Autodesk Inventor part; units mm, degrees
ref_plane "YZ Plane" through (0, 0, 0) normal (1, 0, 0) x (0, 1, 0)
ref_plane "XZ Plane" through (0, 0, 0) normal (0, 1, 0) x (-1, 0, 0)
ref_plane "XY Plane" through (0, 0, 0) normal (0, 0, 1) x (1, 0, 0)
sketch "Sketch1" plane through (0, 0, 0) normal (0, 0, 1) x (1, 0, 0)
  circle A0 centre (0, 0) radius 6.5
  dimension "d0" = 13
extrude "Extrusion1" add sketch "Sketch1" along normal blind 2.5
sketch "Sketch2" plane through (0, 0, 2.5) normal (0, 0, 1) x (1, 0, 0)
  circle A0 centre (0, 0) radius 1.55
  dimension "d3" = 3.1
extrude "Extrusion2" cut sketch "Sketch2" against normal through all
sketch "Sketch3" plane through (0, 0, 0) normal (0, 0, -1) x (-1, 0, 0)
  circle A0 centre (0, 0) radius 2.96
  circle A1 centre (0, 0) radius 7.5
  dimension "d6" = 5.92
  dimension "d16" = 15
extrude "Extrusion3" cut sketch "Sketch3" against normal blind 0.8
sketch "Sketch4" plane through (0, 0, 2.5) normal (0, 0, 1) x (1, 0, 0)
  circle A0 centre (0, 0) radius 2.5
  dimension "d9" = 5
extrude "Extrusion4" cut sketch "Sketch4" against normal blind 1.5
sketch "Sketch5" plane through (0, 0, 2.5) normal (0, 0, 1) x (1, 0, 0)
  circle A0 centre (0, 0) radius 6.5
  circle A1 centre (0, 0) radius 2.5
  circle A2 centre (0, 0) radius 3.025
  circle A3 centre (0, 0) radius 6.5
  dimension "d12" = 6.05
  dimension "d15" = 0
extrude "Extrusion5" add sketch "Sketch5" along normal blind 2.5 contours A0
chamfer "Chamfer1" distance 2 angle 45 1 edges at (-6.5, 0, 0.8)
properties part number "motor_and_magnet_holder"
Work out the finished part from the listing and answer in its coordinate system (mm). A direction names the side the tool comes from. Round coordinates to 2 decimals unless told otherwise and drop trailing zeros. Write each loop counter-clockwise with the first axis right and the second up, starting at its lowest first coordinate (ties: lowest second). Pieces come first, ordered by that corner, then holes. Notation, with made-up numbers: (-20.75, 10.5) -> (21.25, 10.5) arc R26 cw to (21.25, 40.5) -> close; hole circle Ø3 at (-32.75, -25). An arc over 180 degrees is marked (long way). Write each question's results on one line, items separated by ' | '.
Item 1: Which of the six approach directions +Z, -Z, +X, -X, +Y, -Y give full straight-line access (tool end or side, diameter ignored) to faces 4 (the face through (-2, 2, 2.5)), 5 (the face through (-5.158, 3.955, 3.885)), 6 (the face through (2.35, -1.8, 0.39))?
Result set:
face 4: +Z | face 5: +Z, -Z | face 6: -Z
Item 2: A cutting plane is placed at A-A, the plane y = 0. Determine the outline of the cut face in (x, z) (3 decimals), plus the area to 3 significant figures.
Result set:
outline: (-6.5, 2.8) -> (-4.5, 0.8) -> (-2.96, 0.8) -> (-2.96, 0) -> (-1.55, 0) -> (-1.55, 1) -> (-2.5, 1) -> (-2.5, 2.5) -> (-3.025, 2.5) -> (-3.025, 5) -> (-6.5, 5) -> close; (1.55, 0) -> (2.96, 0) -> (2.96, 0.8) -> (4.5, 0.8) -> (6.5, 2.8) -> (6.5, 5) -> (3.025, 5) -> (3.025, 2.5) -> (2.5, 2.5) -> (2.5, 1) -> (1.55, 1) -> close | area: 29.6 mm^2
Item 3: A cutting plane is placed at C-C, the plane z = 1.75. Determine the outline of the cut face in (x, y).
Result set:
outline: circle Ø10.9 at (0, 0); hole circle Ø5 at (0, 0)
Item 4: Flat-ended cylindrical pins translate along their axes: P1, Ø1.8, axis at x = 0, y = -1.5, coming from the +Z side; P2, Ø2.5, axis at x = -1, y = -0.5, coming from the -Z side; P3, Ø1.5, axis at x = 4, y = -0.5, coming from the -Z side; P4, Ø2, axis at y = 4, z = 0.5, coming from the -X side. Find the tip coordinate at first contact, or state that the pin passes through.
Result set:
P1: z = 1 | P2: z = 0 | P3: z = 0.8 | P4: x = -3.67
Item 5: Find the intervals of material crossed by line 1 along Y through (x, z) = (0, 0.3); line 2 along X through (y, z) = (-5.75, 3.75); line 3 along Z through (x, y) = (-1, 3), in increasing order. Write a range as [from, to].
Result set:
line 1: [-2.96, -1.55], [1.55, 2.96] | line 2: [-3.03, 3.03] | line 3: [0.8, 5]
Item 6: The mould has two halves that part along X. Classify faces 1 (the face through (1.3, -1.3, 0)), 2 (the face through (-0.6, 4.59, 0.93)), 3 (the face through (2, 0, 1)): +X half, -X half, draft (parallel to the pull), parting line (faces both ways), or undercut.
Result set:
face 1: draft | face 2: parting line | face 3: undercut
